Geometry: see drawing. Coordinates: mm, zero at the bounding-box minimum. A direction names the side the tool comes from. Give positions to 0.01 mm unless a question says otherwise; leave off trailing zeros. Write each loop counter-clockwise with the first axis right and the second up, starting at its lowest first coordinate (ties: lowest second). Pieces come first, ordered by that corner, then holes. Notation, with made-up numbers: (48, 56.25) - (58, 56.25) arc R26 ccw to (58, 87.25) - close; hole circle Ø11 at (-13.5, -16). An arc over 180 degrees is marked (long way). One line per question, with ' | ' between items. Start each with the question number.
(1) Access query for the marked faces 4, 5 and 6. Directions: +Z, -Z, +X, -X, +Y, -Y. A direction counts if a zero-diameter tool reaches every point of the face in a straight line with its end or side. Return the directions, or none.
(2) Ray query, line 1 (Y direction, x = 6, z = 1.7); line 2 (X direction, y = 4, z = 54.1) (1 decimal); line 3 (X direction, y = 1.75, z = 29) (1 decimal). Return the intervals inside material, ascending. Write a range as [from, to].
(3) Draft query along Z for the marked faces 1, 2 and 3. Return one class per face: +Z half, -Z half, draft (parallel to the pull), parting line (faces both ways), or undercut.
(4) Section B-B, the plane x = 6. Return loops of the section in (y, z).
(5) Section A-A, the plane z = 19. Return loops of the section in (x, y) (1 decimal), plus the area to 3 significant figures.
(6) Section C-C, the plane z = 29. Return loops of the section in (x, y) (1 decimal).
(7) Section D-D, the plane y = 4. State how many separate pieces and enclosed holes the cut face has, plus the area to 3 significant figures.
(8) Pin query (flat end, axial travel): pin 1 (2 mm diameter, centred on y = 3, z = 6.5, fed in from +X) (1 decimal); pin 2 (10 mm diameter, centred on x = 35.5, z = 31.5, fed in from +Y); pin 3 (2.5 mm diameter, centred on y = 4, z = 23.5, fed in from +X); pin 4 (4 mm diameter, centred on y = 3, z = 26.5, fed in from -X). Return the tip coordinate at first contact, or that it passes through.
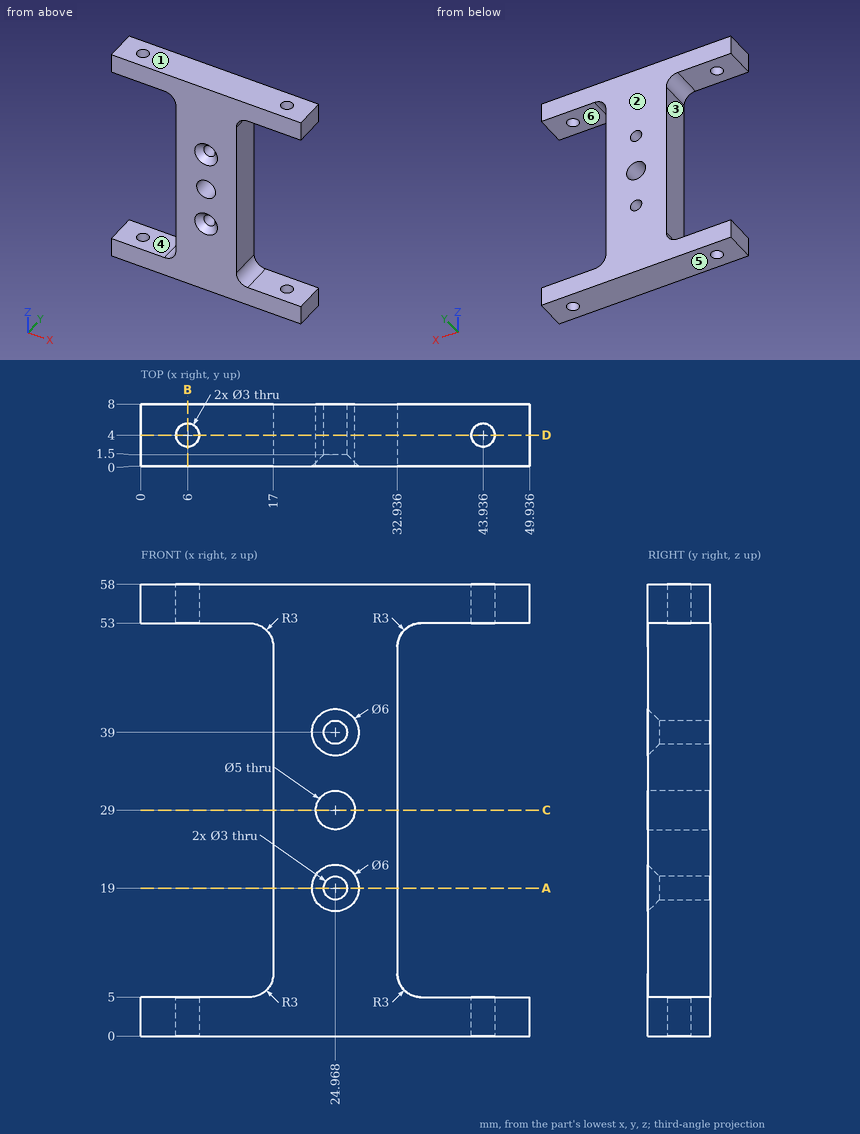
Check sheet entries:
1) face 4: -X, +Y, -Y | face 5: -Z, +X, -X, +Y, -Y | face 6: +X, +Y, -Y
2) line 1: [0, 2.5], [5.5, 8] | line 2: [0, 4.5], [7.5, 42.4], [45.4, 49.9] | line 3: [17, 22.5], [27.5, 32.9]
3) face 1: +Z half | face 2: draft | face 3: undercut
4) outline: (0, 0) - (2.5, 0) - (2.5, 5) - (0, 5) - close; (0, 53) - (2.5, 53) - (2.5, 58) - (0, 58) - close; (5.5, 0) - (8, 0) - (8, 5) - (5.5, 5) - close; (5.5, 53) - (8, 53) - (8, 58) - (5.5, 58) - close
5) outline: (17, 0) - (22, 0) - (23.5, 1.5) - (23.5, 8) - (17, 8) - close; (26.5, 1.5) - (28, 0) - (32.9, 0) - (32.9, 8) - (26.5, 8) - close | area: 101 mm²
6) outline: (17, 0) - (22.5, 0) - (22.5, 8) - (17, 8) - close; (27.5, 0) - (32.9, 0) - (32.9, 8) - (27.5, 8) - close
7) separate pieces: 5 | enclosed holes: 3 | area: 1,180 mm²
8) pin 1: x = 34.3 | pin 2: y = 8 | pin 3: x = 32.94 | pin 4: x = 17
